Read the model definition and answer for the solid it produces. Units are mm, in the model's axes. A direction names the side the tool comes from. Give positions to 0.01 mm unless a question says otherwise; leave off trailing zeros. Order: outer loops, then holes, each group sorted by start corner. A loop starts at its lowest first (then second) coordinate and runs counter-clockwise, first axis right, second up.
Autodesk Inventor part; units mm, degrees
ref_plane "YZ Plane" through (0, 0, 0) normal (1, 0, 0) x (0, 1, 0)
ref_plane "XZ Plane" through (0, 0, 0) normal (0, 1, 0) x (-1, 0, 0)
ref_plane "XY Plane" through (0, 0, 0) normal (0, 0, 1) x (1, 0, 0)
sketch "Sketch1" plane through (0, 0, 0) normal (0, 1, 0) x (-1, 0, 0)
  circle A0 centre (0, 0) radius 4
  circle A1 centre (0, 0) radius 10
  circle A2 centre (-16, 0) radius 2.75
  line L0 (21.5, -4) -> (-21.5, -4)
  line L1 (-21.5, -4) -> (-21.5, 4)
  line L2 (-21.5, 4) -> (21.5, 4)
  line L3 (21.5, 4) -> (21.5, -4)
  line L4 (21.5, -4) -> (-21.5, 4) construction
  line L5 (-21.5, -4) -> (21.5, 4) construction
  line L6 (21.5, 0) -> (-21.5, 0)
  circle A3 centre (16, 0) radius 2.75
  line L7 (0, 10) -> (0, -14)
  line L8 (-21.5, 4) -> (-2.8689, 9.5796)
  line L9 (21.5, 4) -> (2.8689, 9.5796)
  line L10 (21.5, -4) -> (2.8689, -9.5796)
  line L11 (-21.5, -4) -> (-2.8689, -9.5796)
  line L12 (-10, -14) -> (10, -14)
  line L13 (10, -14) -> (10, -4)
  line L14 (10, 0) -> (-10, 0)
  line L15 (-10, -4) -> (-10, -14)
  dimension "d0" = 8
  dimension "d1" = 20
  dimension "d2" = 5.5
  dimension "d3" = 43
  dimension "d4" = 8
  dimension "d5" = 16
  dimension "d6" = 5.5
  dimension "d7" = 16
  dimension "d8" = 24
  dimension "d9" = 0
  dimension "d10" = 10
extrude "Extrusion1" add sketch "Sketch1" along normal blind 5 contours L6 A1 L0 A0 | A0 L2 A1 L6 | A0 L6 A1 L2 | L7 A1 L2 | L2 A1 L7 | L0 A1 L6 A0 | L7 A1 L0 | L0 A1 L7 | L6 A3 L3 L0 A1 | A1 L2 L3 L6 A3 | L2 L8 A1 | A1 L6 A2 L1 L2 | A1 L9 L2 | L0 L13 L10 A1 | L0 L1 L6 A2 A1 | A1 L11 L15 L0 | L7 L12 L15 L11 A1 | A1 L10 L13 L12 L7 | L0 L10 L13 | L15 L11 L0
sketch "Sketch2" plane through (0, 5, 0) normal (0, 1, 0) x (1, 0, 0)
  circle A0 centre (0, 0) radius 4
  arc A1 (-10, 0) -> (10, 0) centre (0, 0) ccw
  line L0 (-10, 14) -> (10, 14)
  line L1 (10, 14) -> (10, 0)
  line L2 (-10, 0) -> (-10, 14)
  circle A2 centre (0, 0) radius 4
  dimension "d13" = 20
  dimension "d15" = 20
extrude "Extrusion2" add sketch "Sketch2" along normal blind 5
properties part number "shf8"
1) For a pull along X with two mould halves and no side action, classify faces 4 (the face through (-13.253, 2.465, -0.121)), 5 (the face through (-15.83, 2.46, -5.7)), 6 (the face through (15.83, 2.46, -5.7)), 7 (the face through (18.747, 2.465, -0.121)) as released by +X, released by -X, zero draft, split by the parting line, or undercut.
Final values:
face 4: undercut
face 5: released by -X
face 6: released by +X
face 7: undercut
2) A tool of negligible diameter and unlimited length cuts with its end or side. For faces 1 (the face through (10, 6, -9)), 2 (the face through (-10, 6, -8)), 3 (the face through (0, 7, 10)), from which of +Z, -Z, +X, -X, +Y, -Y can it reach the whole face along a straight path? Write none if from no direction.
Final values:
face 1: -Z, +X, +Y
face 2: -Z, -X, +Y
face 3: +Z, +Y
3) Given pin 1 (9 mm diameter, centred on x = 16, z = 0, fed in from +Y); pin 2 (4.5 mm diameter, centred on x = -16, z = 0, fed in from +Y); pin 3 (1.5 mm diameter, centred on y = 8.5, z = 0.5, fed in from -X), each flat-ended and moving along its own axis, determine where each tip first touches the part or whether it passes through.
Final values:
pin 1: stops at y = 5
pin 2: passes through
pin 3: stops at x = -10
4) Consider L1, parallel to X at y = 2.25, z = 0; L2, parallel to Z at x = 0, y = 2.15; L3, parallel to X at y = 2.25, z = 1.5. Determine where each line is inside the solid, lowest interval first.
Final values:
L1: x = -21.5 to -18.75, -13.25 to -4, 4 to 13.25, 18.75 to 21.5
L2: z = -14 to -4, 4 to 10
L3: x = -21.5 to -18.3, -13.7 to -3.71, 3.71 to 13.7, 18.3 to 21.5
5) The part is cut by section D-D on z = 5. Determine the outline of the cut face in (x, y).
Final values:
outline: (-18.16, 0) - (18.16, 0) - (18.16, 5) - (8.66, 5) - (8.66, 10) - (-8.66, 10) - (-8.66, 5) - (-18.16, 5) - close
6) The part is cut by section B-B on x = 0. Determine the outline of the cut face in (y, z), and give its area (3 significant figures).
Final values:
outline: (0, -14) - (10, -14) - (10, -4) - (0, -4) - close; (0, 4) - (10, 4) - (10, 10) - (0, 10) - close
area: 160 mm2
7) The part is cut by section C-C on y = 6. Determine the outline of the cut face in (x, z), and give its area (3 significant figures).
Final values:
outline: (-10, -14) - (10, -14) - (10, 0) arc R10 ccw to (-10, 0) - close; hole circle Ø8 at (0, 0)
area: 387 mm2
8) The part is cut by section A-A on y = 2. Determine the outline of the cut face in (x, z).
Final values:
outline: (-21.5, -4) - (-10, -7.44) - (-10, -14) - (10, -14) - (10, -7.44) - (21.5, -4) - (21.5, 4) - (2.87, 9.58) arc R10 ccw to (-2.87, 9.58) - (-21.5, 4) - close; hole circle Ø5.5 at (-16, 0); hole circle Ø8 at (0, 0); hole circle Ø5.5 at (16, 0)
